Verification items for the finished model (mm, model axes). Face numbers are marked on the shaded views. A direction names the side the tool comes from. Give positions to 0.01 mm unless a question says otherwise; leave off trailing zeros. Order: outer loops, then holes, each group sorted by start corner. A loop starts at its lowest first (then second) coordinate and runs counter-clockwise, first axis right, second up.
(1) Scan lines: L1, parallel to Y at x = 0, z = 1.25; L2, parallel to Z at x = 26, y = 19.5; L3, parallel to Y at x = -52.5, z = -0.25. Record each from-to range of solid material in increasing order.
(2) Gauge pin test, flat ends, axial feed: pin 1 (5 mm diameter, centred on x = -17.5, y = 15.5, fed in from -Z); pin 2 (3 mm diameter, centred on y = 3.5, z = -2, fed in from +X); pin 3 (3 mm diameter, centred on x = 24.5, z = -2.5, fed in from +Y); pin 4 (1.5 mm diameter, centred on x = -49, z = -1.5, fed in from +Y). Record the tip position at first contact, or that the pin passes through.
(3) Sectioned sample at B-B on y = -15.5. Record the cut outline in (x, z), plus the area to 3 significant figures.
(4) Mould release check, pull along X, two halves, no side actions. Record for the marked faces 3, 4 and 5: pulls with the +X half, pulls with the -X half, needs draft (parallel to the pull), parting line crosses it, or undercut.
(5) Sectioned sample at C-C on z = -4.5. Count the separate pieces of the cut face and the enclosed holes in it, plus the area to 3 significant figures.
(6) Access from +Z, -Z, +X, -X, +Y, -Y to the whole of each face (thin tool, end or side, straight path). Record for the marked faces 1 and 2.
(7) Sectioned sample at D-D on x = -26. Record the cut outline in (y, z), plus the area to 3 significant figures.
(8) Sectioned sample at A-A on x = 0. Record the cut outline in (y, z).
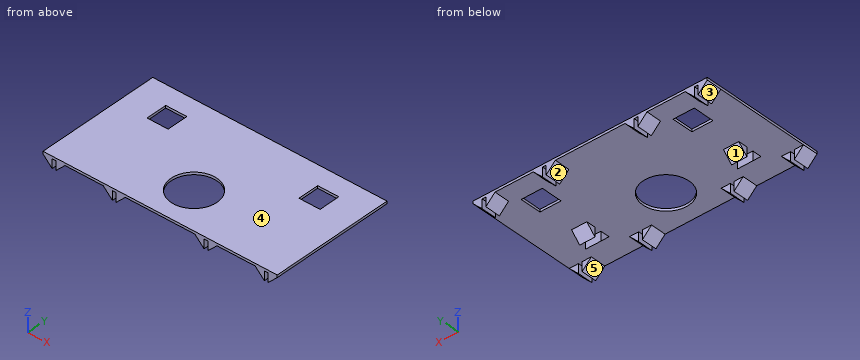
```python
from build123d import *

# Parameters (mm, degrees)
F2_DEPTH  = 81
F3_DEPTH  = 10
F4_START  = -71
F4_DEPTH  = 10
F7_DEPTH  = 5
F9_R      = 15
F10_DEPTH = 1.6
F11_W     = 13.8
F11_H     = 13.8
F12_DEPTH = 1.6


# Not quite as in the source:
# - a feature names something its author has since deleted; it is built from what else it names


with BuildPart() as f2:
    # F1 (on offset) → F2 (new body)
    with BuildSketch(Plane.XZ.offset(40.5)):
        Polygon((76.55, 0), (76.55, 1.6), (-76.55, 1.6), (-76.55, 0), (-70.55, 0), (-68.15, 0), (-62.15, 0), (-37.15, 0), (-31.15, 0), (-28.75, 0), (-22.75, 0), (22.75, 0), (28.75, 0), (31.15, 0), (37.15, 0), (62.15, 0), (68.15, 0), (70.55, 0), align=None)
    extrude(amount=-F2_DEPTH)

    # F1 (on offset) → F3 (join)
    with BuildSketch(Plane.XZ.offset(40.5)):
        Polygon((-62.15, 0), (-68.15, 0), (-68.15, -6), align=None)
        Polygon((-31.15, 0), (-37.15, 0), (-31.15, -6), align=None)
        Polygon((-22.75, 0), (-28.75, 0), (-28.75, -6), align=None)
        Polygon((-70.55, 0), (-76.55, 0), (-70.55, -6), align=None)
    extrude(amount=-F3_DEPTH)

    # F1 (on offset) → F4 (join)
    with BuildSketch(Plane.XZ.offset(40.5).offset(F4_START)):
        Polygon((-62.15, 0), (-68.15, 0), (-68.15, -6), align=None)
        Polygon((-31.15, 0), (-37.15, 0), (-31.15, -6), align=None)
        Polygon((-22.75, 0), (-28.75, 0), (-28.75, -6), align=None)
        Polygon((-70.55, 0), (-76.55, 0), (-70.55, -6), align=None)
    extrude(amount=-F4_DEPTH)

    # F6 (on offset) → F7 (join, symmetric)
    with BuildSketch(Plane.YZ.offset(-49.65)):
        Polygon((-13.5, 0), (-13.5, -6), (-7.5, 0), align=None)
        Polygon((-17.9, -6), (-17.9, 0), (-23.9, 0), align=None)
    extrude(amount=F7_DEPTH, both=True)

    # F8: F2 across plane


with BuildPart() as f2_1:
    add(f2.part)
    add(f2.part.mirror(Plane.YZ))

    # F9 (on face) → F10 (cut)
    with BuildSketch(Plane.XY.offset(1.6)):
        with Locations((0, -15.5)):
            Circle(F9_R)
    extrude(amount=-F10_DEPTH, mode=Mode.SUBTRACT)

    # F11 (on face) → F12 (cut)
    with BuildSketch(Plane.XY.offset(1.6)):
        with Locations((-49.65, 20.6)):
            Rectangle(F11_W, F11_H)
        with Locations((49.65, 20.6)):
            Rectangle(F11_W, F11_H)
    extrude(amount=-F12_DEPTH, mode=Mode.SUBTRACT)


solid = f2_1.part
```
Ans:
1. L1: y = -40.5 to -30.5, -0.5 to 40.5
1. L2: z = 0 to 1.6
1. L3: y = -23.65 to -17.9, -13.5 to -7.75
2. pin 1: stops at z = 0
2. pin 2: passes through
2. pin 3: stops at y = 40.5
2. pin 4: stops at y = -8.25
3. outline: (-76.55, 0) - (-15, 0) - (-15, 1.6) - (-76.55, 1.6) - close; (15, 0) - (76.55, 0) - (76.55, 1.6) - (15, 1.6) - close
3. area: 197 mm2
4. face 3: pulls with the -X half
4. face 4: needs draft
4. face 5: undercut
5. separate pieces: 20
5. enclosed holes: 0
5. area: 300 mm2
6. face 1: -Z, +X, -X, +Y
6. face 2: -Z, +Y, -Y
7. outline: (-40.5, -3.25) - (-30.5, -3.25) - (-30.5, 0) - (30.5, 0) - (30.5, -3.25) - (40.5, -3.25) - (40.5, 1.6) - (-40.5, 1.6) - close
7. area: 195 mm2
8. outline: (-40.5, 0) - (-30.5, 0) - (-30.5, 1.6) - (-40.5, 1.6) - close; (-0.5, 0) - (40.5, 0) - (40.5, 1.6) - (-0.5, 1.6) - close
